Input: part model. Units: mm. Frame: model coordinates. Face numbers are marked on the shaded views. Coordinates: 2 decimals unless noted, no trailing zeros. Write each loop counter-clockwise with the first axis right and the second up, starting at its lowest first coordinate (ties: lowest second). Pieces come first, ordered by that corner, then holes. Notation, with made-up numbers: (85, 85.5) - (126, 85.5) arc R21 cw to (126, 109.5) - close; hole circle Ø6 at (72.25, 33.25). An arc over 180 degrees is marked (long way). Use a Markdown table: item, result. Add a question column.
Q1. Section query C-C (y = 15.5). Return the cut outline in (x, z).
Q2. Material intervals for probe 1 along Z at (x, y) = (-10, 12.5); probe 2 along X at (y, z) = (4.5, 57); probe 3 along Z at (x, y) = (-10, 4.5), sorted ascending. Write a range as from..to.
Q3. Mould query, pull axis Z, two halves, no side actions, for the marked faces 1, 2 and 3. Classes: released by +Z, released by -Z, zero draft, split by the parting line, or undercut.
Q4. Section query D-D (x = -89.5). Return the cut outline in (y, z), then the cut area to 3 significant figures.
Q5. Section query B-B (x = -10). Return the cut outline in (y, z), then the cut area to 4 significant figures.
Q6. Section query A-A (z = 101.75). Return the cut outline in (x, y), then the cut area to 3 significant figures.
Q7. Pin query (flat end, axial travel): P1, Ø8, axis at x = -5.5, z = 6, coming from the -Y side; P2, Ø12, axis at y = 16, z = 94.5, coming from the +X side; P3, Ø3, axis at y = 5, z = 6.5, coming from the +X side. Return the tip coordinate at first contact, or that it passes through.
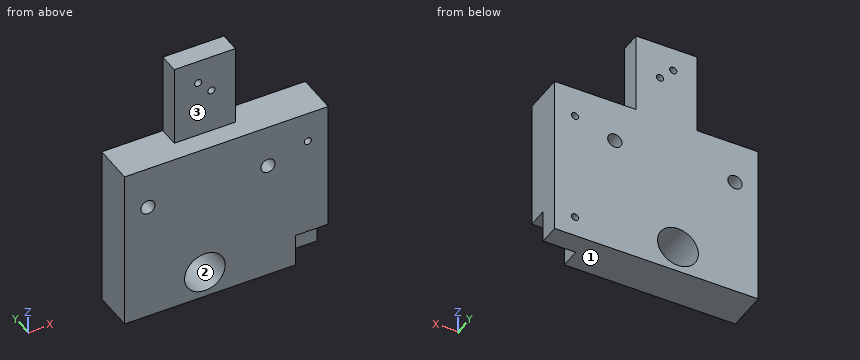
Autodesk Inventor part; units mm, degrees
ref_plane "YZ Plane" through (0, 0, 0) normal (1, 0, 0) x (0, 1, 0)
ref_plane "XZ Plane" through (0, 0, 0) normal (0, 1, 0) x (-1, 0, 0)
ref_plane "XY Plane" through (0, 0, 0) normal (0, 0, 1) x (1, 0, 0)
sketch "Boceto1" plane through (0, 0, 0) normal (0, 1, 0) x (-1, 0, 0)
  line L0 (100, 80) -> (-100, 80)
  line L1 (-100, 80) -> (-100, -80)
  line L2 (-100, -80) -> (100, -80)
  line L3 (100, -80) -> (100, 80)
  line L4 (100, 80) -> (-100, -80) construction
  line L5 (-100, 80) -> (100, -80) construction
  point P0 (0, 0)
  dimension "d0" = 200
  dimension "d1" = 160
extrude "Extrusión1" add sketch "Boceto1" along normal blind 20
sketch "Boceto2" plane through (0, 20, 0) normal (0, 1, 0) x (1, 0, 0)
  line L0 (-100, 80) -> (-100, -80)
  line L1 (-100, 80) -> (-70, 80)
  line L2 (-70, 80) -> (-70, 40)
  line L3 (-70, 40) -> (-100, 40)
  line L4 (-100, 40) -> (-100, 80)
  line L5 (100, 80) -> (-100, 80)
  line L6 (0, 80) -> (0, 40)
  line L7 (100, 80) -> (70, 80)
  line L8 (70, 80) -> (70, 40)
  line L9 (70, 40) -> (100, 40)
  line L10 (100, 40) -> (100, 80)
  point P0 (0, 0)
  dimension "d4" = 30
  dimension "d5" = 40
extrude "Extrusión2" cut sketch "Boceto2" against normal blind 10
sketch "Boceto3" plane through (0, 20, 0) normal (0, 1, 0) x (1, 0, 0)
  line L0 (-70, 80) -> (-70, 40)
  line L1 (-70, 80.0001) -> (-70, 40)
  line L2 (-70, 40) -> (-100, 40)
  line L3 (-100, 40) -> (-100, 80.0001)
  line L4 (-100, 40) -> (-70, 40)
  line L5 (-70, 40) -> (-70, 80)
  line L6 (-70, 80) -> (-100, 80)
  line L7 (-100, 80) -> (-100, 40)
  circle A0 centre (-88.25, 58.25) radius 1.75
  circle A1 centre (-81.75, 51.75) radius 1.75
  line L8 (100, 80) -> (-100, 80)
  line L9 (0, 80) -> (0, 56.5)
  circle A2 centre (88.25, 58.25) radius 1.75
  circle A3 centre (81.75, 51.75) radius 1.75
  point P0 (0, 0)
  point P1 (-64.3507, 80)
  point P2 (-74.3507, 0)
  point P3 (-85, 80)
  dimension "d23" = 21.75
  dimension "d24" = 11.75
  dimension "d26" = 11.75
hole "Agujero1" at (-81.75, 20, -51.75) at (-88.25, 20, -58.25) at (81.75, 20, -51.75) at (88.25, 20, -58.25) direction (0, -1, 0) diameter 3.5 end through all
sketch "Boceto4" plane through (-100, 0, 80) normal (0, 0, 1) x (1, 0, 0)
  line L0 (30, 20) -> (60, 20)
  line L1 (60, 20) -> (60, 10)
  line L2 (60, 10) -> (30, 10)
  line L3 (30, 10) -> (30, 20)
  line L4 (0, 0) -> (0, 20)
  line L5 (100, 0) -> (100, 10)
  line L6 (170, 20) -> (140, 20)
  line L7 (140, 20) -> (140, 10)
  line L8 (140, 10) -> (170, 10)
  line L9 (170, 10) -> (170, 20)
  dimension "d34" = 30
  dimension "d35" = 10
  dimension "d36" = 30
extrude "Extrusión3" add sketch "Boceto4" along normal blind 40
sketch "Boceto5" plane through (0, 20, 0) normal (0, 1, 0) x (1, 0, 0)
  line L0 (59.9999, -50) -> (69.9999, -50)
  line L1 (49.9999, -101.75) -> (49.9999, -79.9497)
  line L2 (59.9999, -108.25) -> (59.9999, -50)
  line L3 (40, -80) -> (69.9999, -80)
  line L4 (49.9999, -79.9497) -> (40, -80)
  circle A0 centre (51.7499, -101.75) radius 1.75
  circle A1 centre (58.2499, -108.25) radius 1.75
  line L5 (69.9999, -80) -> (69.9999, -120)
  line L6 (40, -120) -> (40, -80)
  line L7 (69.9999, -120) -> (40, -120)
  line L8 (0, -50) -> (0, -71.75)
  line L9 (-40, -120) -> (-40, -80)
  line L10 (-49.9999, -101.75) -> (-49.9999, -79.9497)
  circle A2 centre (-51.7499, -101.75) radius 1.75
  circle A3 centre (-58.2499, -108.25) radius 1.75
  line L11 (-40, -80) -> (-69.9999, -80)
  line L12 (-69.9999, -120) -> (-40, -120)
  line L13 (-69.9999, -80) -> (-69.9999, -120)
  line L14 (-59.9999, -108.25) -> (-59.9999, -50)
  line L15 (-40, -120) -> (-69.9999, -120)
  line L16 (-69.9999, -80) -> (-69.9999, -120)
  line L17 (-40, -120) -> (-70, -120)
  line L18 (-40, -80) -> (-40, -120)
  line L19 (-59.9999, -110) -> (-49.9999, -110)
  line L20 (-49.9999, -110) -> (-49.9999, -100)
  line L21 (-49.9999, -100) -> (-59.9999, -100)
  line L22 (-59.9999, -100) -> (-59.9999, -110)
  line L23 (-100, 40) -> (-100, -80)
  point P0 (0, 0)
  point P1 (-56.75, -68.25)
  point P2 (-63.25, -61.75)
  point P3 (63.25, -61.75)
  point P4 (56.75, -68.25)
  dimension "d45" = 3.5
  dimension "d46" = 3.5
  dimension "d39" = 10
  dimension "d40" = 10
  dimension "d41" = 40
  dimension "d42" = 0
  dimension "d43" = 6.5
  dimension "d44" = 6.5
  dimension "d47" = 11.7499
  dimension "d48" = 11.75
  dimension "d49" = 0
  dimension "d50" = 11.75
  dimension "d51" = 0
  dimension "d97" = 40.0001
hole "Agujero2" at (-58.2499, 20, 108.25) at (-51.7499, 20, 101.75) at (51.7499, 20, 101.75) at (58.2499, 20, 108.25) direction (0, -1, 0) diameter 3.5 end through all
sketch "Boceto6" plane through (0, 20, 0) normal (0, 1, 0) x (1, 0, 0)
  circle A0 centre (-60.569, -13.1067) radius 10
  circle A1 centre (-29.569, -59.1067) radius 3.5
  line L0 (-60.569, -13.1067) -> (-39.0083, -13.1067)
  circle A2 centre (-29.569, 25.8933) radius 3.5
  circle A3 centre (-88.569, 25.8933) radius 3.5
  circle A4 centre (-88.569, -59.1067) radius 3.5
  line L1 (70.4544, -63.0517) -> (18.4544, -63.0517)
  line L2 (18.4544, -63.0517) -> (18.4544, 6.9483)
  line L3 (18.4544, 6.9483) -> (70.4544, 6.9483)
  line L4 (70.4544, 6.9483) -> (70.4544, -63.0517)
  line L5 (70.4544, 6.9483) -> (48.4544, 6.9483)
  line L6 (48.4544, 6.9483) -> (48.4544, 48.9483)
  line L7 (48.4544, 48.9483) -> (70.4544, 48.9483)
  line L8 (70.4544, 48.9483) -> (70.4544, 6.9483)
  line L9 (77.2288, -8.158) -> (77.2281, -5.6604)
  circle A5 centre (63.7706, -5.7606) radius 1.75
  line L10 (70.7641, -24.1464) -> (70.7641, 22.2796)
  circle A6 centre (35.8307, -5.7609) radius 1.75
  line L11 (25.1581, -13.2381) -> (25.1581, -10.7404)
  circle A7 centre (68.8507, -57.8309) radius 1.75
  line L12 (26.4277, 35.0051) -> (26.4277, 37.5029)
  circle A8 centre (20.6074, -56.5614) radius 1.75
  line L13 (18.6941, -55.9176) -> (70.7641, -55.9176)
  line L14 (18.6941, -55.9176) -> (18.6941, -7.6743)
  line L15 (44.7291, -55.9176) -> (44.7291, -31.7959)
  line L16 (63.7706, -28.0517) -> (26.4277, -28.0517)
  line L17 (44.7291, -23.5247) -> (44.7291, -31.7959)
  point P0 (0, 0)
  point P1 (-60.569, -16.6067)
  point P2 (45.425, 12.8886)
  point P3 (44.7291, -28.0517)
  dimension "d59" = 7
  dimension "d60" = 7
  dimension "d61" = 7
  dimension "d62" = 39
  dimension "d63" = 46
  dimension "d64" = 59
  dimension "d65" = 46
  dimension "d66" = 39
  dimension "d67" = 59
  dimension "d68" = 52
  dimension "d69" = 70
  dimension "d70" = 22
  dimension "d71" = 42
  dimension "d72" = 3.5
  dimension "d73" = 3.5
  dimension "d74" = 3.5
  dimension "d75" = 3.5
  dimension "d142" = 17.3763
  dimension "d143" = 12.7092
  dimension "d144" = 6.6837
  dimension "d145" = 12.7089
  dimension "d146" = 5.2208
  dimension "d147" = 1.6037
  dimension "d148" = 2.1531
  dimension "d149" = 6.4903
hole "Agujero3" at (68.8507, 20, 57.8309) at (20.6074, 20, 56.5614) at (63.7706, 20, 5.7606) at (35.8307, 20, 5.7609) direction (0, -1, 0) diameter 3.5 end through all
sketch "Boceto7" plane through (0, 20, 0) normal (0, 1, 0) x (1, 0, 0)
  circle A0 centre (-60.569, -13.1067) radius 10
  circle A1 centre (-29.569, -59.1067) radius 3.5
  line L0 (-60.569, -13.1067) -> (-39.0083, -13.1067)
  circle A2 centre (-29.569, 25.8933) radius 3.5
  circle A3 centre (-88.569, 25.8933) radius 3.5
  circle A4 centre (-88.569, -59.1067) radius 3.5
  point P0 (0, 0)
  point P1 (-60.569, -16.6067)
  dimension "d83" = 7
  dimension "d84" = 7
  dimension "d85" = 7
  dimension "d86" = 39
  dimension "d87" = 46
  dimension "d88" = 59
  dimension "d89" = 46
  dimension "d90" = 39
  dimension "d91" = 59
extrude "Extrusión4" cut sketch "Boceto7" against normal blind 20
ref_plane "Plano de trabajo1" through (0, 0, -80) normal (-1, 0, 0) x (0, 0, 1)
ref_plane "Plano de trabajo2" through (100, 0, 0) normal (0, 0, -1) x (-1, 0, 0)
sketch "Boceto8" plane through (0, 20, 0) normal (0, 1, 0) x (1, 0, 0)
  line L0 (80, -15) -> (90, -15)
  circle A0 centre (85, -10) radius 1.75
  line L1 (85, 10) -> (85, -10)
  line L2 (90, -15) -> (90, 15)
  circle A1 centre (85, 10) radius 1.75
  line L3 (80, 15) -> (80, -15)
  line L4 (90, 15) -> (80, -15) construction
  line L5 (80, 15) -> (90, -15) construction
  line L6 (90, 15) -> (80, 15)
  line L7 (100, -80) -> (100, 40)
  line L8 (0, 0) -> (20, -20)
  line L9 (0, 0) -> (28.2843, 0) construction
  line L10 (15, -60) -> (15, -70)
  circle A2 centre (10, -65) radius 1.75
  line L11 (-10, -65) -> (10, -65)
  line L12 (15, -70) -> (-15, -70)
  circle A3 centre (-10, -65) radius 1.75
  line L13 (-15, -60) -> (15, -60)
  line L14 (-15, -70) -> (15, -60) construction
  line L15 (-15, -60) -> (15, -70) construction
  line L16 (-15, -70) -> (-15, -60)
  line L17 (0, 0) -> (18.6615, 18.6615)
  line L18 (0, 0) -> (26.3913, 0) construction
  line L19 (-15, 60) -> (-15, 70)
  circle A4 centre (-10, 65) radius 1.75
  line L20 (10, 65) -> (-10, 65)
  line L21 (-15, 70) -> (15, 70)
  circle A5 centre (10, 65) radius 1.75
  line L22 (15, 60) -> (-15, 60)
  line L23 (15, 70) -> (-15, 60) construction
  line L24 (15, 60) -> (-15, 70) construction
  line L25 (15, 70) -> (15, 60)
  line L26 (70, 80) -> (-70, 80)
  line L27 (-40, -80) -> (40, -80)
  point P0 (86.9608, 0)
  point P1 (86.9608, 0)
  point P2 (85, 15)
  point P3 (0, -69.1269)
  point P4 (0, -69.1269)
  point P5 (-15, -67.1661)
  point P6 (0, 69.7066)
  point P7 (0, 69.7066)
  point P8 (15, 67.7458)
  point P9 (-15, 65)
  point P10 (15, -65)
  dimension "d98" = 10
  dimension "d99" = 30
  dimension "d100" = 10
  dimension "d101" = 5
  dimension "d102" = 5
  dimension "d103" = 5
  dimension "d104" = 5
  dimension "d105" = 45
  dimension "d106" = 45
  dimension "d107" = 10
  dimension "d108" = 10
  dimension "d109" = 30
  dimension "d110" = 5
  dimension "d111" = 5
  dimension "d112" = 5
  dimension "d113" = 5
  dimension "d114" = 10
  dimension "d115" = 30
  dimension "d116" = 5
  dimension "d117" = 5
  dimension "d118" = 5
  dimension "d119" = 5
  dimension "d120" = 10
hole "Agujero4" at (-10, 20, -65) at (10, 20, -65) at (85, 20, -10) at (85, 20, 10) at (10, 20, 65) at (-10, 20, 65) direction (0, -1, 0) diameter 3.5 end through all
sketch "Boceto9" plane through (0, 20, 0) normal (0, 1, 0) x (1, 0, 0)
  circle A0 centre (10, -10) radius 1.75
  line L0 (6.803, 0) -> (14.6069, 0)
  line L1 (0, 0) -> (0, -4.8284)
  line L2 (0, 0) -> (20.0354, 0)
  circle A1 centre (10, 10) radius 1.75
  line L3 (0, 0) -> (0, 4.8284)
  circle A2 centre (-10, 10) radius 1.75
  circle A3 centre (-10, -10) radius 1.75
  dimension "d128" = 3.5
  dimension "d129" = 10
  dimension "d130" = 10
hole "Agujero5" at (-10, 20, 10) at (-10, 20, -10) at (10, 20, -10) at (10, 20, 10) direction (0, -1, 0) diameter 3.5 end through all
sketch "Boceto10" plane through (0, 0, 0) normal (0, -1, 0) x (1, 0, 0)
  line L0 (-16, 16) -> (16, 16)
  line L1 (16, 16) -> (16, -16)
  line L2 (16, -16) -> (-16, -16)
  line L3 (-16, -16) -> (-16, 16)
  line L4 (-16, 16) -> (16, -16) construction
  line L5 (16, 16) -> (-16, -16) construction
  point P0 (0, 0)
  point P1 (0, 0)
  dimension "d138" = 32
  dimension "d139" = 32
extrude "Extrusión5" cut sketch "Boceto10" against normal blind 10
split "Dividir1" plane through (100, 0, 0) removes the side toward (0, 0, -1)
split "Dividir2" plane through (0, 0, -80) removes the side toward (1, 0, 0)
properties part number "base_mid_3"
Values follow:
| question | item | result |
|---|---|---|
| 1 | outline | (-100, 0) - (0, 0) - (0, 80) - (-40, 80) - (-40, 120) - (-70, 120) - (-70, 80) - (-100, 80) - close; hole circle Ø7 at (-88.57, 59.11); hole circle Ø20 at (-60.57, 13.11); hole circle Ø3.5 at (-58.25, 108.25); hole circle Ø3.5 at (-51.75, 101.75); hole circle Ø7 at (-29.57, 59.11); hole circle Ø3.5 at (-10, 10); hole circle Ø3.5 at (-10, 65) |
| 2 | probe 1 | 0..8.25, 11.75..63.25, 66.75..80 |
| 2 | probe 2 | -100..-91.36, -85.77..-32.36, -26.77..0 |
| 2 | probe 3 | 16..63.25, 66.75..80 |
| 3 | face 1 | released by -Z |
| 3 | face 2 | undercut |
| 3 | face 3 | zero draft |
| 4 | outline | (0, 0) - (20, 0) - (20, 55.73) - (0, 55.73) - close; (0, 62.48) - (20, 62.48) - (20, 80) - (0, 80) - close |
| 4 | area | 1,470 mm2 |
| 5 | outline | (0, 16) - (10, 16) - (10, 11.75) - (20, 11.75) - (20, 63.25) - (0, 63.25) - close; (0, 66.75) - (20, 66.75) - (20, 80) - (0, 80) - close; (10, 0) - (20, 0) - (20, 8.25) - (10, 8.25) - close |
| 5 | area | 1,335 mm2 |
| 6 | outline | (-70, 10) - (-53.5, 10) - (-53.5, 20) - (-70, 20) - close; (-50, 10) - (-40, 10) - (-40, 20) - (-50, 20) - close |
| 6 | area | 265 mm2 |
| 7 | P1 | y = 10 |
| 7 | P2 | x = -40 |
| 7 | P3 | x = -16 |
